```python
from build123d import *

# Parameters (mm, degrees)
SKETCH1_W           = 40
SKETCH1_H           = 60
BOSS_EXTRUDE1_DEPTH = 10
SKETCH2_W           = 5.4
SKETCH2_H           = 5.4
CUT_EXTRUDE1_DEPTH  = 38.416573868
SKETCH3_W           = 60
SKETCH3_H           = 6
BOSS_EXTRUDE2_DEPTH = 30
CUT_EXTRUDE2_DEPTH  = 47.904157598
FILLET2_R           = 1
FILLET3_R           = 5


with BuildPart() as part:
    # Sketch1 → Boss-Extrude1 (new body)
    with BuildSketch(Plane(origin=(0, 0, 0), x_dir=(0, 1, 0), z_dir=(0, 0, 1))):
        Rectangle(SKETCH1_W, SKETCH1_H)
    extrude(amount=BOSS_EXTRUDE1_DEPTH)

    # Sketch2 → Cut-Extrude1 (cut, through all)
    with BuildSketch(Plane.XY.offset(10)):
        with Locations((-17.35, 10.3)):
            Rectangle(SKETCH2_W, SKETCH2_H)
        with Locations((17.35, 10.3)):
            Rectangle(SKETCH2_W, SKETCH2_H)
    extrude(amount=-CUT_EXTRUDE1_DEPTH, mode=Mode.SUBTRACT)

    # Sketch3 → Boss-Extrude2 (add)
    with BuildSketch(Plane.XY.offset(10)):
        with Locations((0, -17)):
            Rectangle(SKETCH3_W, SKETCH3_H)
    extrude(amount=BOSS_EXTRUDE2_DEPTH)

    # Sketch4 → Cut-Extrude2 (cut, through all)
    with BuildSketch(Plane.XY.offset(10)):
        Polygon((-24, 1.6), (-8.65, 1.6), (-8.65, 14), (8.65, 14), (8.65, 1.6), (24, 1.6), (24, -10), (-24, -10), align=None)
    extrude(amount=-CUT_EXTRUDE2_DEPTH, mode=Mode.SUBTRACT)

    # Fillet2
    fillet2_edges = [part.edges().sort_by_distance(p)[0] for p in [
        (-24, -10, 5),
        (-24, 1.6, 5),
        (-8.65, 1.6, 5),
        (-8.65, 14, 5),
        (8.65, 14, 5),
        (8.65, 1.6, 5),
        (24, 1.6, 5),
        (24, -10, 5),
    ]]
    fillet(fillet2_edges, radius=FILLET2_R)

    # Fillet3
    fillet3_edges = [part.edges().sort_by_distance(p)[0] for p in [
        (30, -20, 20),
        (-30, -20, 20),
    ]]
    fillet(fillet3_edges, radius=FILLET3_R)


solid = part.part
```
The listing builds one solid part. Answer for the finished solid, in the listing's coordinates (mm). A direction names the side the tool comes from. Coordinates: 2 decimals unless noted, no trailing zeros. Order: outer loops, then holes, each group sorted by start corner. A loop starts at its lowest first (then second) coordinate and runs counter-clockwise, first axis right, second up. Notation, with made-up numbers: M -16,-4 L 17,-4 A17 ccw 17,13 Z; hole C -27.5,51 d9. An arc over 180 degrees is marked long. Answer as a JSON object with one key per item and string values. Group by question number.
1. Straight lines are drawn through the part: line 1 (X direction, y = 8, z = 6.5); line 2 (X direction, y = -6, z = 4); line 3 (Y direction, x = -4.5, z = 3.5). For each, find the intervals that lie inside material, in ascending order.
2. Section B-B on x = 3 is taken. Write down the section's boundary in (y, z).
3. Determine the mould class of faces 1 (the flat face through (17, 7.6, 5)), 2 (the flat face through (-30, 1, 8)), 3 (the cylindrical face through (29, -18, 20)) for opening direction Y: released by +Y, released by -Y, zero draft, split by the parting line, or undercut.
4. Section C-C on y = 4.5 is taken. Write down the section's boundary in (x, z), then the cut area to 3 significant figures.
5. Section A-A on y = -8 is taken. Write down the section's boundary in (x, z).
6. Flat-ended cylindrical pins translate along their axes: P1, Ø1, axis at x = -10.5, z = 32, coming from the +Y side; P2, Ø10, axis at x = 15, y = -2.5, coming from the +Z side. Find the tip coordinate at first contact, or state that the pin passes through.
7. Section D-D on z = 27 is taken. Write down the section's boundary in (x, y).
8. A tool of negligible diameter and unlimited length cuts with its end or side. For faces 4 (the flat face through (0, 18, 10)), 5 (the flat face through (0, -14, 0)), 6 (the flat face through (8.65, 8, 5)), from which of +Z, -Z, +X, -X, +Y, -Y can it reach the whole face along a straight path? Write none if from no direction.
Values follow:
{
 "1": {"line 1": "-30 to -20.05, -14.65 to -8.65, 8.65 to 14.65, 20.05 to 30", "line 2": "-30 to -24, 24 to 30", "line 3": "-20 to -10, 14 to 20"},
 "2": {"outline": "M -20,0 L -10,0 L -10,10 L -14,10 L -14,40 L -20,40 Z; M 14,0 L 20,0 L 20,10 L 14,10 Z"},
 "3": {"face 1": "undercut", "face 2": "zero draft", "face 3": "released by -Y"},
 "4": {"outline": "M -30,0 L -8.65,0 L -8.65,10 L -30,10 Z; M 8.65,0 L 30,0 L 30,10 L 8.65,10 Z", "area": "427 mm2"},
 "5": {"outline": "M -30,0 L -24,0 L -24,10 L -30,10 Z; M 24,0 L 30,0 L 30,10 L 24,10 Z"},
 "6": {"P1": "y = -14", "P2": "z = 10"},
 "7": {"outline": "M -30,-15 A5 ccw -25,-20 L 25,-20 A5 ccw 30,-15 L 30,-14 L -30,-14 Z"},
 "8": {"face 4": "+Z, +X, -X, +Y", "face 5": "-Z, +X, -X, +Y, -Y", "face 6": "+Z, -Z"}
}
